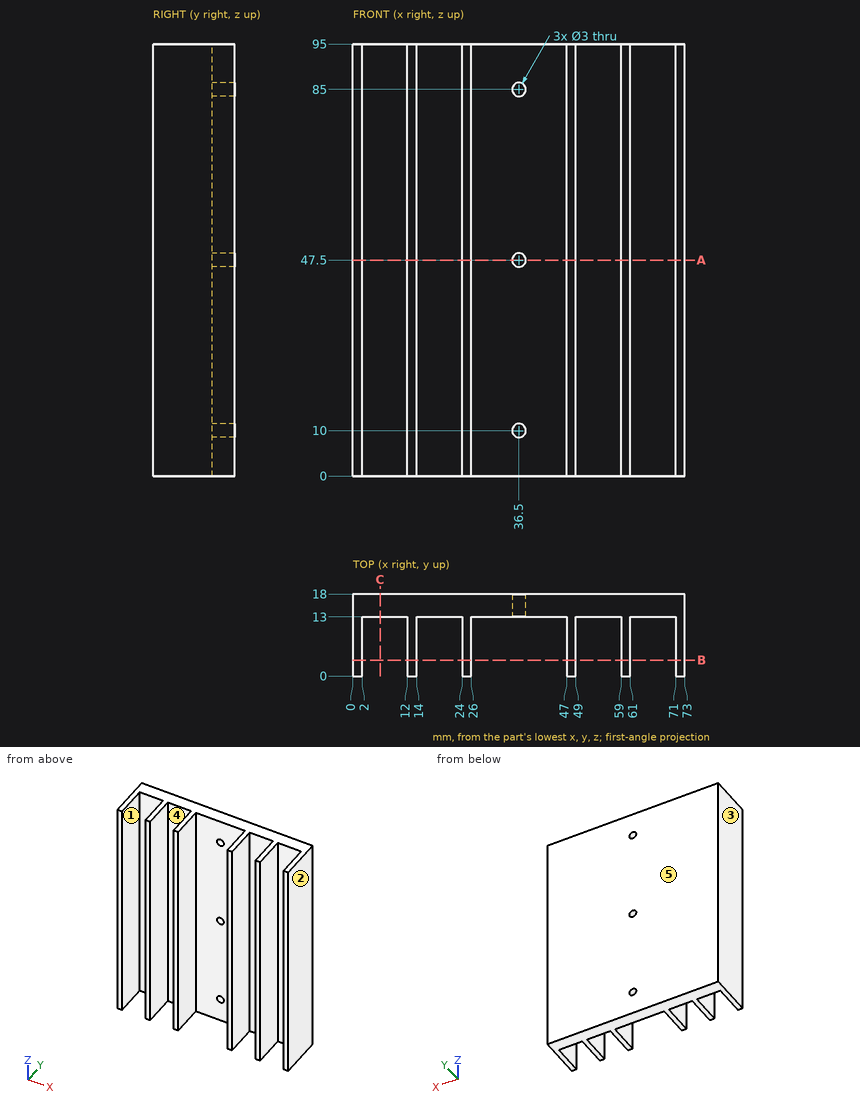
Drawing for the job (mm, zero at the part's lowest x, y, z). A direction names the side the tool comes from. Round coordinates to 2 decimals unless told otherwise and drop trailing zeros. Loops run counter-clockwise (first coordinate to the right, second up) from the corner with the lowest first, then second, coordinate; pieces in that order, holes last. Notation, with made-up numbers: M 82.5,50.25 L 111.5,50.25 A15 ccw 111.5,67.25 Z; hole C 38,57.5 d10. An arc over 180 degrees is marked long. Use a Markdown table: item, result. Add a question column.
(1) Cut at A-A (z = 47.5). Give the cut face in (x, y).
(2) Cut at C-C (x = 6). Give the cut face in (y, z), and give its area (3 significant figures).
(3) Which spindle directions (+Z, -Z, +X, -X, +Y, -Y) get a long thin tool onto all of the face, cutting with end or side? Do the marked faces 4 and 5. Say none if no direction does.
(4) Cut at B-B (y = 3.5). Give the cut face in (x, z), and give its area (3 significant figures).
(5) Pull direction X, two halves, no side cores. Call the marked faces 1, 2 and 3: +X half, -X half, draft (parallel to the pull), parting line (faces both ways), or undercut.
(6) Flat gauge pin, fed straight in: pin 1 (6.5 mm diameter, centred on x = 38, z = 53.5, fed in from -Y). Where does the tip first touch, or does it go through?
(7) Drill centre lines: line 1 (X direction, y = 5.5, z = 34); line 2 (Z direction, x = 36.5, y = 16); line 3 (Y direction, x = 44, z = 81). Where is each one in solid material? Low to high.
Geometry says:
| question | item | result |
|---|---|---|
| 1 | outline | M 0,0 L 2,0 L 2,13 L 12,13 L 12,0 L 14,0 L 14,13 L 24,13 L 24,0 L 26,0 L 26,13 L 35,13 L 35,18 L 0,18 Z; M 38,13 L 47,13 L 47,0 L 49,0 L 49,13 L 59,13 L 59,0 L 61,0 L 61,13 L 71,13 L 71,0 L 73,0 L 73,18 L 38,18 Z |
| 2 | outline | M 13,0 L 18,0 L 18,95 L 13,95 Z |
| 2 | area | 475 mm² |
| 3 | face 4 | +Z, -Z, -Y |
| 3 | face 5 | +Z, -Z, +X, -X, +Y |
| 4 | outline | M 0,0 L 2,0 L 2,95 L 0,95 Z; M 12,0 L 14,0 L 14,95 L 12,95 Z; M 24,0 L 26,0 L 26,95 L 24,95 Z; M 47,0 L 49,0 L 49,95 L 47,95 Z; M 59,0 L 61,0 L 61,95 L 59,95 Z; M 71,0 L 73,0 L 73,95 L 71,95 Z |
| 4 | area | 1,140 mm² |
| 5 | face 1 | undercut |
| 5 | face 2 | +X half |
| 5 | face 3 | -X half |
| 6 | pin 1 | stops at y = 13 |
| 7 | line 1 | x = 0 to 2, 12 to 14, 24 to 26, 47 to 49, 59 to 61, 71 to 73 |
| 7 | line 2 | z = 0 to 8.5, 11.5 to 46, 49 to 83.5, 86.5 to 95 |
| 7 | line 3 | y = 13 to 18 |
